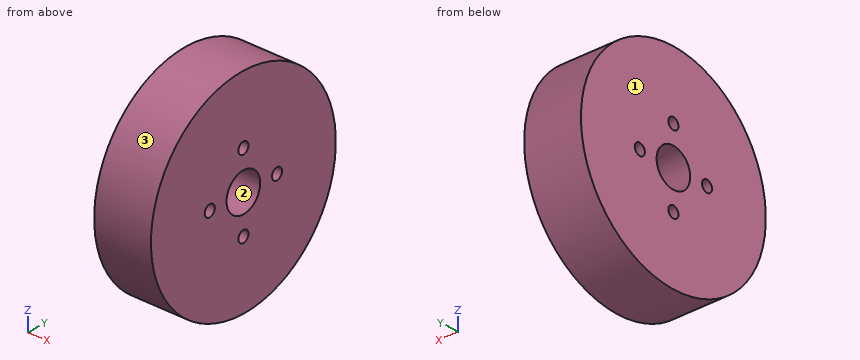
from build123d import *

# Parameters (mm, degrees)
SKETCH_1_R          = 27.5
EXTRUDE_1_DEPTH     = 15
CUT_EXTRUDE_1_REACH = 65.997
SKETCH_2_R          = 5
SKETCH_2_R_2        = 1.5


with BuildPart() as part:
    # 草图1 → 凸台-拉伸1 (new body)
    with BuildSketch(Plane(origin=(0, 0, 0), x_dir=(0, 0, -1), z_dir=(1, 0, 0))):
        with Locations((-18.795257752, 14.06192285)):
            Circle(SKETCH_1_R)
    extrude(amount=EXTRUDE_1_DEPTH)

    # 草图2 → 切除-拉伸1 (cut, up to next)
    with BuildSketch(Plane.ZY, mode=Mode.PRIVATE) as cut_extrude_1_sk1:
        with Locations((18.795257752, 14.06192285)):
            Circle(SKETCH_2_R)
    cut_extrude_1_tool1 = extrude(cut_extrude_1_sk1.sketch, amount=-CUT_EXTRUDE_1_REACH, mode=Mode.PRIVATE) & part.part
    # 草图2 → 切除-拉伸1 (cut, up to next)
    with BuildSketch(Plane.ZY, mode=Mode.PRIVATE) as cut_extrude_1_sk2:
        with Locations((18.795257752, 24.06192285)):
            Circle(SKETCH_2_R_2)
    cut_extrude_1_tool2 = extrude(cut_extrude_1_sk2.sketch, amount=-CUT_EXTRUDE_1_REACH, mode=Mode.PRIVATE) & part.part
    # 草图2 → 切除-拉伸1 (cut, up to next)
    with BuildSketch(Plane.ZY, mode=Mode.PRIVATE) as cut_extrude_1_sk3:
        with Locations((28.795257752, 14.06192285)):
            Circle(SKETCH_2_R_2)
    cut_extrude_1_tool3 = extrude(cut_extrude_1_sk3.sketch, amount=-CUT_EXTRUDE_1_REACH, mode=Mode.PRIVATE) & part.part
    # 草图2 → 切除-拉伸1 (cut, up to next)
    with BuildSketch(Plane.ZY, mode=Mode.PRIVATE) as cut_extrude_1_sk4:
        with Locations((8.795257752, 14.06192285)):
            Circle(SKETCH_2_R_2)
    cut_extrude_1_tool4 = extrude(cut_extrude_1_sk4.sketch, amount=-CUT_EXTRUDE_1_REACH, mode=Mode.PRIVATE) & part.part
    # 草图2 → 切除-拉伸1 (cut, up to next)
    with BuildSketch(Plane.ZY, mode=Mode.PRIVATE) as cut_extrude_1_sk5:
        with Locations((18.795257752, 4.06192285)):
            Circle(SKETCH_2_R_2)
    cut_extrude_1_tool5 = extrude(cut_extrude_1_sk5.sketch, amount=-CUT_EXTRUDE_1_REACH, mode=Mode.PRIVATE) & part.part
    add(cut_extrude_1_tool1.solids().sort_by_distance((0, 14.061923, 18.795258))[0], mode=Mode.SUBTRACT)
    add(cut_extrude_1_tool2.solids().sort_by_distance((0, 24.061923, 18.795258))[0], mode=Mode.SUBTRACT)
    add(cut_extrude_1_tool3.solids().sort_by_distance((0, 14.061923, 28.795258))[0], mode=Mode.SUBTRACT)
    add(cut_extrude_1_tool4.solids().sort_by_distance((0, 14.061923, 8.795258))[0], mode=Mode.SUBTRACT)
    add(cut_extrude_1_tool5.solids().sort_by_distance((0, 4.061923, 18.795258))[0], mode=Mode.SUBTRACT)


solid = part.part
Part model, mm, in its own coordinate system. Face numbers are marked on the shaded views. Give positions to 0.01 mm unless a question says otherwise; leave off trailing zeros. Loops run counter-clockwise (first coordinate to the right, second up) from the corner with the lowest first, then second, coordinate; pieces in that order, holes last. Notation, with made-up numbers: (5.25, 50) -> (23.25, 50) arc R16 cw to (23.25, 61) -> close; hole circle Ø9 at (17.25, 11.5). An arc over 180 degrees is marked (long way). Write each question's results on one line, items separated by ' | '. Start each with the question number.
Q1. Pin check, flat tips, straight feed: P1, Ø2.5, axis at y = 4.06, z = 18.8, coming from the +X side; P2, Ø8, axis at x = 3.5, z = 26, coming from the +Y side; P3, Ø3, axis at x = 10, y = 30, coming from the -Z side; P4, Ø6, axis at x = 9, z = 28, coming from the +Y side. Stop position of each tip, or through.
Q2. Band-saw the part on A-A on y = 10. List the corners of the cut face in (x, z), plus the area to 3 significant figures.
Q3. Band-saw the part on B-B on x = 2.5. List the corners of the cut face in (y, z).
Q4. Band-saw the part on C-C on z = 11. List the corners of the cut face in (x, y).
Q5. Wall check: L1, parallel to Y at x = 12.5, z = 18; L2, parallel to Y at x = 5, z = 20; L3, parallel to Z at x = 10.25, y = 15. Give the ranges that are in metal, low to high.
Q6. Band-saw the part on D-D on y = 27. List the corners of the cut face in (x, z), plus the area to 3 significant figures.
Q7. Pull direction Y, two halves, no side cores. Call the marked faces 1, 2 and 3: +Y half, -Y half, draft (parallel to the pull), parting line (faces both ways), or undercut.
Results are:
1) P1: passes through | P2: stops at y = 41.37 | P3: stops at z = -4.61 | P4: stops at y = 40.85
2) outline: (0, -8.4) -> (15, -8.4) -> (15, 15.88) -> (0, 15.88) -> close; (0, 21.71) -> (15, 21.71) -> (15, 45.99) -> (0, 45.99) -> close | area: 728 mm²
3) outline: circle Ø55 at (14.06, 18.8); hole circle Ø3 at (4.06, 18.8); hole circle Ø10 at (14.06, 18.8); hole circle Ø3 at (14.06, 8.8); hole circle Ø3 at (14.06, 28.8); hole circle Ø3 at (24.06, 18.8)
4) outline: (0, -12.31) -> (15, -12.31) -> (15, 40.43) -> (0, 40.43) -> close
5) L1: y = -13.43 to 2.79, 5.33 to 9.13, 19 to 22.79, 25.33 to 41.55 | L2: y = -13.41 to 3.17, 4.96 to 9.21, 18.91 to 23.17, 24.96 to 41.54 | L3: z = -8.69 to 7.62, 9.97 to 13.88, 23.71 to 27.62, 29.97 to 46.28
6) outline: (0, -5.47) -> (15, -5.47) -> (15, 43.06) -> (0, 43.06) -> close | area: 728 mm²
7) face 1: draft | face 2: undercut | face 3: parting line
